Source: CAD feature listing. Evaluate the final solid. Frame: model axes, mm. A direction names the side the tool comes from. Coordinates: 2 decimals unless noted, no trailing zeros. Order: outer loops, then holes, each group sorted by start corner. A loop starts at its lowest first (then second) coordinate and runs counter-clockwise, first axis right, second up.
Item 1: Section B-B on y = 0. State how many separate pieces and enclosed holes the cut face has, then the cut area to 4 significant figures.
Item 2: Ray query, line 1 (Y direction, x = -1.5, z = 8.25); line 2 (Y direction, x = 6, z = 13); line 3 (Y direction, x = 34, z = 11.75). Return the intervals inside material, ascending.
Item 3: Contact query for flat-ended pins moving along their axis: P1, Ø2, axis at x = -45, z = 12, coming from the +Y side; P2, Ø3, axis at y = -30, z = 9, coming from the -X side; P3, Ø1.5, axis at y = -24, z = 7, coming from the -X side; P4, Ø5, axis at x = 21, y = 38, coming from the -Z side. Output: stop coordinate, or through.
Item 4: Section C-C on x = 0. Return the cut outline in (y, z), then the cut area to 3 significant figures.
Item 5: Section D-D on y = -33.5. Return the cut outline in (x, z), then the cut area to 3 significant figures.
Item 6: Reachability of faces 1 (the cylindrical face through (-39.987, 0.572, 9.535)), 2 (the cylindrical face through (-14.303, -9.736, 5.479)), 3 (the cylindrical face through (-13.17, 4.36, 13.52)) from +Z, -Z, +X, -X, +Y, -Y: full face, straight path, thin tool, end or side. Return the list, or none.
Item 7: Section A-A on x = -36. Return the cut outline in (y, z), then the cut area to 3 significant figures.
Item 8: Mould query, pull axis Y, two halves, no side actions, for faces 4 (the flat face through (-24, 16, 4)), 5 (the cylindrical face through (-12.68, -57.11, 7.4)), 6 (the flat face through (39, 39, 15)). Classes: released by +Y, released by -Y, zero draft, split by the parting line, or undercut.
from build123d import *

# Parameters (mm, degrees)
SKETCH1_R           = 58.5
BOSS_EXTRUDE1_DEPTH = 15
SKETCH2_R           = 55
SKETCH2_R_2         = 49.25
CUT_EXTRUDE1_DEPTH  = 10
SKETCH3_R           = 11.75
CUT_EXTRUDE2_DEPTH  = 85.080318743
SKETCH4_R           = 16.25
CUT_EXTRUDE3_DEPTH  = 7
SKETCH5_R           = 19.5
CUT_EXTRUDE4_DEPTH  = 4
SKETCH6_R           = 16
CUT_EXTRUDE5_DEPTH  = 3
SKETCH7_R           = 14.5
CUT_EXTRUDE6_DEPTH  = 3
SKETCH8_R           = 13
CUT_EXTRUDE7_DEPTH  = 84.597248759


with BuildPart() as part:
    # Sketch1 → Boss-Extrude1 (new body)
    with BuildSketch(Plane.XY):
        Circle(SKETCH1_R)
    extrude(amount=BOSS_EXTRUDE1_DEPTH)

    # Sketch2 → Cut-Extrude1 (cut)
    with BuildSketch(Plane.XY.offset(15)):
        Circle(SKETCH2_R)
        Circle(SKETCH2_R_2, mode=Mode.SUBTRACT)
    extrude(amount=-CUT_EXTRUDE1_DEPTH, mode=Mode.SUBTRACT)

    # Sketch3 → Cut-Extrude2 (cut, through all)
    with BuildSketch(Plane(origin=(0, 0, 0), x_dir=(-1, 0, 0), z_dir=(0, 0, -1))):
        with Locations((-25, 0)):
            Circle(SKETCH3_R)
    extrude(amount=-CUT_EXTRUDE2_DEPTH, mode=Mode.SUBTRACT)

    # Sketch4 → Cut-Extrude3 (cut)
    with BuildSketch(Plane.XY.offset(15)):
        with Locations((25, 0)):
            Circle(SKETCH4_R)
    extrude(amount=-CUT_EXTRUDE3_DEPTH, mode=Mode.SUBTRACT)

    # Sketch5 → Cut-Extrude4 (cut)
    with BuildSketch(Plane(origin=(0, 0, 0), x_dir=(-1, 0, 0), z_dir=(0, 0, -1))):
        with Locations((27, 0)):
            Circle(SKETCH5_R)
    extrude(amount=-CUT_EXTRUDE4_DEPTH, mode=Mode.SUBTRACT)

    # Sketch6 → Cut-Extrude5 (cut)
    with BuildSketch(Plane(origin=(0, 0, 4), x_dir=(-1, 0, 0), z_dir=(0, 0, -1))):
        with Locations((27, 0)):
            Circle(SKETCH6_R)
    extrude(amount=-CUT_EXTRUDE5_DEPTH, mode=Mode.SUBTRACT)

    # Sketch7 → Cut-Extrude6 (cut)
    with BuildSketch(Plane.XY.offset(15)):
        with Locations((-27, 0)):
            Circle(SKETCH7_R)
    extrude(amount=-CUT_EXTRUDE6_DEPTH, mode=Mode.SUBTRACT)

    # Sketch8 → Cut-Extrude7 (cut, through all)
    with BuildSketch(Plane.XY.offset(12)):
        with Locations((-27, 0)):
            Circle(SKETCH8_R)
    extrude(amount=-CUT_EXTRUDE7_DEPTH, mode=Mode.SUBTRACT)


solid = part.part
Answer list:
1. separate pieces: 3
1. enclosed holes: 0
1. area: 755.5 mm2
2. line 1: y = -58.48 to -54.98, -49.23 to 49.23, 54.98 to 58.48
2. line 2: y = -58.19 to -54.67, -48.88 to 48.88, 54.67 to 58.19
2. line 3: y = -47.61 to -43.23, -35.63 to -13.53, 13.53 to 35.63, 43.23 to 47.61
3. P1: stops at y = 38.55
3. P2: stops at x = -51.09
3. P3: stops at x = -53.68
3. P4: stops at z = 0
4. outline: (-58.5, 0) - (58.5, 0) - (58.5, 15) - (55, 15) - (55, 5) - (49.25, 5) - (49.25, 15) - (-49.25, 15) - (-49.25, 5) - (-55, 5) - (-55, 15) - (-58.5, 15) - close
4. area: 1,640 mm2
5. outline: (-47.96, 0) - (47.96, 0) - (47.96, 15) - (43.62, 15) - (43.62, 5) - (36.1, 5) - (36.1, 15) - (-36.1, 15) - (-36.1, 5) - (-43.62, 5) - (-43.62, 15) - (-47.96, 15) - close
5. area: 1,290 mm2
6. face 1: +Z, -Z
6. face 2: -Z
6. face 3: +Z
7. outline: (-46.11, 0) - (-17.3, 0) - (-17.3, 4) - (-13.23, 4) - (-13.23, 7) - (-9.38, 7) - (-9.38, 12) - (-11.37, 12) - (-11.37, 15) - (-33.61, 15) - (-33.61, 5) - (-41.58, 5) - (-41.58, 15) - (-46.11, 15) - close; (9.38, 7) - (13.23, 7) - (13.23, 4) - (17.3, 4) - (17.3, 0) - (46.11, 0) - (46.11, 15) - (41.58, 15) - (41.58, 5) - (33.61, 5) - (33.61, 15) - (11.37, 15) - (11.37, 12) - (9.38, 12) - close
7. area: 844 mm2
8. face 4: undercut
8. face 5: split by the parting line
8. face 6: zero draft
